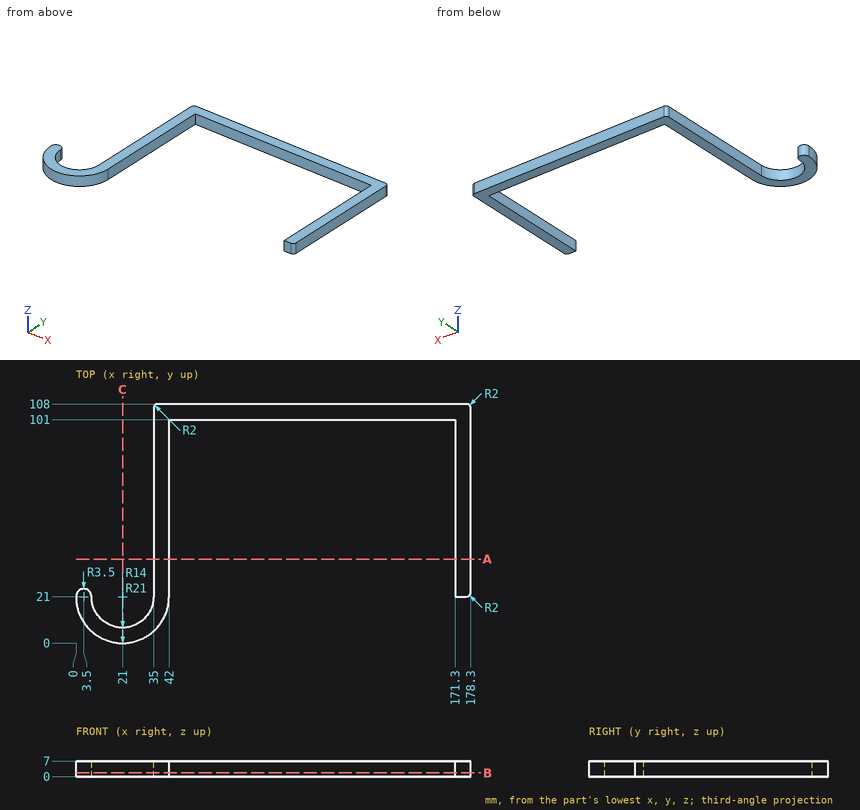
Study the drawing (mm; zero at the part's minimum x, y, z) and answer. Round coordinates to 2 decimals unless told otherwise and drop trailing zeros. Write each loop counter-clockwise with the first axis right and the second up, starting at its lowest first coordinate (ties: lowest second). Pieces come first, ordered by that corner, then holes.
1) A cutting plane is placed at B-B (z = 1.75). Give the vertices of the cut face in (x, y), plus the area to 3 significant figures.
2) Given pin 1 Ø3 at (x, z) = (33.5, 1) entering from -Y; pin 2 Ø3 at (y, z) = (48, 1) entering from -X; pin 3 Ø4 at (x, z) = (173, 4.5) entering from -Y, each flat-ended and moving along its own axis, determine where each tip first touches the part or whether it passes through.
3) A cutting plane is placed at C-C (x = 21). Give the vertices of the cut face in (y, z), plus the area to 3 significant figures.
4) Straight lines are drawn through the part: line 1 (X direction, y = 57, z = 3); line 2 (X direction, y = 23.5, z = 4.25); line 3 (Y direction, x = 142.5, z = 4). For each, find the intervals that lie inside material, in ascending order.
5) A cutting plane is placed at A-A (y = 38). Give the vertices of the cut face in (x, z), plus the area to 3 significant figures.
Completed:
1. outline: (0, 21) arc R21 ccw to (42, 21) - (42, 101) - (171.3, 101) - (171.3, 21) - (176.3, 21) arc R2 ccw to (178.3, 23) - (178.3, 106) arc R2 ccw to (176.3, 108) - (37, 108) arc R2 ccw to (35, 106) - (35, 21) arc R14 cw to (7, 21) arc R3.5 ccw to start
1. area: 2,520 mm2
2. pin 1: stops at y = 3.11
2. pin 2: stops at x = 35
2. pin 3: stops at y = 21
3. outline: (0, 0) - (7, 0) - (7, 7) - (0, 7) - close
3. area: 49.0 mm2
4. line 1: x = 35 to 42, 171.3 to 178.3
4. line 2: x = 1.05 to 5.95, 35 to 42, 171.3 to 178.3
4. line 3: y = 101 to 108
5. outline: (35, 0) - (42, 0) - (42, 7) - (35, 7) - close; (171.3, 0) - (178.3, 0) - (178.3, 7) - (171.3, 7) - close
5. area: 98.0 mm2
